Here's how the part is built. I have some questions about the finished solid (model axes, mm). A direction names the side the tool comes from. Round coordinates to 2 decimals unless told otherwise and drop trailing zeros. Order: outer loops, then holes, each group sorted by start corner. A loop starts at its lowest first (then second) coordinate and runs counter-clockwise, first axis right, second up. Notation, with made-up numbers: (-39.5, 76) - (-18.5, 76) arc R38 cw to (-18.5, 114) - close; hole circle Ø6 at (62.5, 81.25). An arc over 180 degrees is marked (long way). One line per item, written item: value.
from build123d import *

# Parameters (mm, degrees)
SKETCH1_R           = 3
SKETCH1_R_2         = 1.5
BOSS_EXTRUDE1_DEPTH = 6


with BuildPart() as part:
    # Sketch1 → Boss-Extrude1 (new body)
    with BuildSketch(Plane(origin=(0, 0, 0), x_dir=(1, 0, 0), z_dir=(0, 1, 0))):
        Polygon((-72, 72), (-72, 28), (-66, 28), (-66, 4.5), (-62, 4.5), (-62, 6.5), (-59, 6.5), (-59, 4.5), (-56, 4.5), (-56, 1.5), (-59, 1.5), (-59, -0.5), (-62, -0.5), (-62, 1.5), (-66, 1.5), (-66, -22), (-72, -22), (-72, -72), (-22, -72), (-22, -66), (1.5, -66), (1.5, -62), (-0.5, -62), (-0.5, -59), (1.5, -59), (1.5, -56), (4.5, -56), (4.5, -59), (6.5, -59), (6.5, -62), (4.5, -62), (4.5, -66), (28, -66), (28, -72), (72, -72), (72, -22), (78, -22), (78, 28), (72, 28), (72, 72), (28, 72), (28, 78), (-22, 78), (-22, 72), align=None)
        with Locations(Location((3, 3, 0), (0, 0, 270))):
            Circle(SKETCH1_R, mode=Mode.SUBTRACT)
        with Locations(Location((3, 75, 0), (0, 0, 270))):
            Circle(SKETCH1_R_2, mode=Mode.SUBTRACT)
        with Locations(Location((75, 3, 0), (0, 0, 270))):
            Circle(SKETCH1_R_2, mode=Mode.SUBTRACT)
    extrude(amount=BOSS_EXTRUDE1_DEPTH)


solid = part.part
Q1. If I drill on line 1 along X through (y, z) = (3.75, -3); line 2 along X through (y, z) = (5.35, 56.5); line 3 along Z through (x, y) = (75, 1.8), over which ranges is the centre line in solid material (lowest first)?
Results list:
line 1: -56 to 0, 6 to 73.5, 76.5 to 78
line 2: -72 to 1.5, 4.5 to 72
line 3: -28 to -4.5, -1.5 to 22
Q2. Which directions (+Z, -Z, +X, -X, +Y, -Y) give clear straight access to the entire face, cutting with the end or side of a thin tool? Please do faces 4 (the flat face through (-10, 3, 66)), 5 (the flat face through (-69, 3, 22)), 6 (the flat face through (75, 3, -28)).
Results list:
face 4: +Z, +Y, -Y
face 5: -X, +Y, -Y
face 6: -Z, +X, +Y, -Y
Q3. We'd pull the mould along Z, two halves only. Please class faces 1 (the flat face through (16, 3, 66)), 2 (the flat face through (28, 3, -75)), 3 (the cylindrical face through (5.03, 2.96, -5.21)): released by +Z, released by -Z, zero draft, split by the parting line, or undercut.
Results list:
face 1: released by +Z
face 2: zero draft
face 3: undercut
Q4. If we section it at B-B, the plane x = -18.5: Please give me the cut outline in (y, z), then the cut area to 3 significant figures.
Results list:
outline: (0, -78) - (6, -78) - (6, 66) - (0, 66) - close
area: 864 mm²
Q5. If we section it at C-C, the plane z = -68: Please give me the cut outline in (x, y), then the cut area to 3 significant figures.
Results list:
outline: (-72, 0) - (72, 0) - (72, 6) - (-72, 6) - close
area: 864 mm²
Q6. Will these pins go through, and if not, where does the flat tip stop? pin 1 (3 mm diameter, centred on y = 3, z = -76.5, fed in from +X); pin 2 (0.9 mm diameter, centred on x = 3.5, y = 3, fed in from +Z); pin 3 (1 mm diameter, centred on y = 1.5, z = -0.5, fed in from -X).
Results list:
pin 1: x = 28
pin 2: z = 56
pin 3: x = -66
Q7. If we section it at A-A, the plane y = 1.9: Give the number of separate pieces and of enclosed holes in the cut face, then the cut area to 3 significant figures.
Results list:
separate pieces: 1
enclosed holes: 3
area: 20,600 mm²
